Part model, mm, in its own coordinate system. Face numbers are marked on the shaded views. Round coordinates to 2 decimals unless told otherwise and drop trailing zeros. Loops run counter-clockwise (first coordinate to the right, second up) from the corner with the lowest first, then second, coordinate; pieces in that order, holes last.
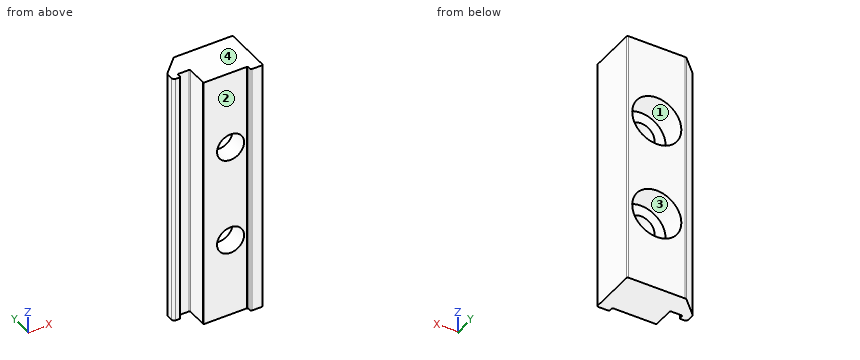
Autodesk Inventor part; units mm, degrees
ref_plane "KLEMMLEISTE_XY" through (-0.25, 0, 0) normal (0, 1, 0) x (1, 0, 0)
ref_plane "KLEMMLEISTE_YZ" through (-0.25, 0, 0) normal (1, 0, 0) x (0, 0, -1)
ref_plane "KLEMMLEISTE_ZX" through (-0.25, 0, 0) normal (0, 0, -1) x (0, 1, 0)
sketch "Sketch_4" plane through (0, 0, 0) normal (0, 0, 1) x (1, 0, 0)
  line L0 (-9.75, 6.2929) -> (-9.75, 5)
  arc A0 (-9.75, 5) -> (-9.25, 4.5) centre (-9.25, 5) ccw
  line L1 (-9.25, 4.5) -> (-8.45, 4.5)
  arc A1 (-8.45, 4.5) -> (-8.25, 4.7) centre (-8.45, 4.7) ccw
  line L2 (-8.25, 4.7) -> (-8.25, 5.3)
  arc A2 (-8.05, 5.5) -> (-8.25, 5.3) centre (-8.05, 5.3) ccw
  line L3 (-8.05, 5.5) -> (-5.95, 5.5)
  arc A3 (-5.75, 5.3) -> (-5.95, 5.5) centre (-5.95, 5.3) ccw
  line L4 (-5.75, 5.3) -> (-5.75, 1.2)
  arc A4 (-5.75, 1.2) -> (-5.55, 1) centre (-5.55, 1.2) ccw
  line L5 (-5.55, 1) -> (3.05, 1)
  arc A5 (3.25, 0.8) -> (3.05, 1) centre (3.05, 0.8) ccw
  line L6 (3.25, 0.8) -> (3.25, 0.2)
  arc A6 (3.25, 0.2) -> (3.45, 0) centre (3.45, 0.2) ccw
  line L7 (3.45, 0) -> (5.55, 0)
  arc A7 (5.55, 0) -> (5.75, 0.2) centre (5.55, 0.2) ccw
  line L8 (5.75, 0.2) -> (5.75, 9.8)
  arc A8 (5.75, 9.8) -> (5.55, 10) centre (5.55, 9.8) ccw
  line L9 (5.55, 10) -> (-6.0429, 10)
  arc A9 (-6.0429, 10) -> (-6.3964, 9.8536) centre (-6.0429, 9.5) ccw
  line L10 (-6.3964, 9.8536) -> (-9.6036, 6.6464)
  arc A10 (-9.6036, 6.6464) -> (-9.75, 6.2929) centre (-9.25, 6.2929) ccw
extrude "Extrusion1" add sketch "Sketch_4" along normal mid plane 52
sketch "Sketch2" plane through (-6.0429, 10, 26) normal (0, 1, 0) x (1, 0, 0)
  point P0 (5.7929, 36)
hole "Hole1" at (-0.25, 10, -10) direction (0, -1, 0) diameter 5.5 depth 10 counterbore diameter 10 counterbore depth 5.2
sketch "Sketch3" plane through (-6.0429, 10, 26) normal (0, 1, 0) x (1, 0, 0)
  point P0 (5.7929, 16)
hole "Hole2" at (-0.25, 10, 10) direction (0, -1, 0) diameter 5.5 depth 10 counterbore diameter 10 counterbore depth 5.2
ref_plane "KLEMMLEISTE_XY" through (-0.25, 0, 0) normal (0, 1, 0) x (1, 0, 0)
ref_plane "KLEMMLEISTE_YZ" through (-0.25, 0, 0) normal (1, 0, 0) x (0, 0, -1)
ref_plane "KLEMMLEISTE_ZX" through (-0.25, 0, 0) normal (0, 0, -1) x (0, 1, 0)
ref_plane "SCHRAUBE_1_XY" through (-0.25, 4.8, -10) normal (0, 1, 0) x (1, 0, 0)
ref_plane "SCHRAUBE_1_YZ" through (-0.25, 4.8, -10) normal (1, 0, 0) x (0, 0, -1)
ref_plane "SCHRAUBE_1_ZX" through (-0.25, 4.8, -10) normal (0, 0, -1) x (0, 1, 0)
ref_plane "SCHRAUBE_2_XY" through (-0.25, 4.8, 10) normal (0, 1, 0) x (1, 0, 0)
ref_plane "SCHRAUBE_2_YZ" through (-0.25, 4.8, 10) normal (1, 0, 0) x (0, 0, -1)
ref_plane "SCHRAUBE_2_ZX" through (-0.25, 4.8, 10) normal (0, 0, -1) x (0, 1, 0)
properties part number "722624 MUE-70/80P1"
1) Slice it at A-A, the plane x = -0.25. Give the cut face in (y, z), then the cut area to 3 significant figures.
Values:
outline: (1, -26) - (10, -26) - (10, -15) - (4.8, -15) - (4.8, -12.75) - (1, -12.75) - close; (1, -7.25) - (4.8, -7.25) - (4.8, -5) - (10, -5) - (10, 5) - (4.8, 5) - (4.8, 7.25) - (1, 7.25) - close; (1, 12.75) - (4.8, 12.75) - (4.8, 15) - (10, 15) - (10, 26) - (1, 26) - close
area: 322 mm2
2) Slice it at D-D, the plane z = 18. Give the cut face in (x, y).
Values:
outline: (-9.75, 5) arc R0.5 ccw to (-9.25, 4.5) - (-8.45, 4.5) arc R0.2 ccw to (-8.25, 4.7) - (-8.25, 5.3) arc R0.2 cw to (-8.05, 5.5) - (-5.95, 5.5) arc R0.2 cw to (-5.75, 5.3) - (-5.75, 1.2) arc R0.2 ccw to (-5.55, 1) - (3.05, 1) arc R0.2 cw to (3.25, 0.8) - (3.25, 0.2) arc R0.2 ccw to (3.45, 0) - (5.55, 0) arc R0.2 ccw to (5.75, 0.2) - (5.75, 9.8) arc R0.2 ccw to (5.55, 10) - (-6.04, 10) arc R0.5 ccw to (-6.4, 9.85) - (-9.6, 6.65) arc R0.5 ccw to (-9.75, 6.29) - close
3) Slice it at C-C, the plane y = 3.75. Give the cut face in (x, z), then the cut area to 3 significant figures.
Values:
outline: (-5.75, -26) - (5.75, -26) - (5.75, 26) - (-5.75, 26) - close; hole circle Ø5.5 at (-0.25, -10); hole circle Ø5.5 at (-0.25, 10)
area: 550 mm2
4) Wall check: line 1 along Z through (x, y) = (-0.25, 2.3); line 2 along Z through (x, y) = (-0.25, 7); line 3 along Y through (x, z) = (-4, 15). Give the ranges that are in metal, low to high.
Values:
line 1: z = -26 to -12.75, -7.25 to 7.25, 12.75 to 26
line 2: z = -26 to -15, -5 to 5, 15 to 26
line 3: y = 1 to 10
5) Drop flat-ended pins along their axis: pin 1 Ø0.5 at (y, z) = (0.5, 5.5) entering from -X; pin 2 Ø0.6 at (x, z) = (-9, 5) entering from -Y; pin 3 Ø1.7 at (x, z) = (-7, 7) entering from -Y. Give the stop position or say it passes through.
Values:
pin 1: stops at x = 3.25
pin 2: stops at y = 4.5
pin 3: stops at y = 5.5
6) Mould opens along Z. For the marked faces 1, 2, 3 and 4 say: released by +Z, released by -Z, zero draft, split by the parting line, or undercut.
Values:
face 1: undercut
face 2: zero draft
face 3: undercut
face 4: released by +Z
